Source: CAD feature listing. Evaluate the final solid. Frame: model axes, mm. Round coordinates to 2 decimals unless told otherwise and drop trailing zeros. Order: outer loops, then holes, each group sorted by start corner. A loop starts at its lowest first (then second) coordinate and runs counter-clockwise, first axis right, second up. Notation, with made-up numbers: (73, 17.25) -> (114, 17.25) arc R21 ccw to (114, 27.25) -> close; hole circle Ø10 at (61, 25). An arc over 180 degrees is marked (long way). Use a Markdown table: item, result. Add a question column.
```python
from build123d import *

# Parameters (mm, degrees)
F0_W     = 300
F0_H     = 10
F1_DEPTH = 100
F2_R     = 2.75
F2_R_2   = 4.25
F3_DEPTH = 10.001
F4_R     = 2.75
F5_DEPTH = 10.001
F6_SIZE  = 0.5


with BuildPart() as f1:
    # F0 (on Right) → F1 (new body)
    with BuildSketch(Plane.YZ):
        with Locations((-150, 5)):
            Rectangle(F0_W, F0_H)
    extrude(amount=F1_DEPTH)

    # F2 (on face) → F3 (cut, through all)
    with BuildSketch(Plane.XY.offset(10)):
        with Locations((60.5, -83)):
            Circle(F2_R)
        with Locations((39.5, -83)):
            Circle(F2_R)
        with Locations((39.5, -217)):
            Circle(F2_R)
        with Locations((60.5, -217)):
            Circle(F2_R)
        with Locations((15, -215)):
            Circle(F2_R_2)
        with Locations((15, -195)):
            Circle(F2_R_2)
        with Locations((15, -83)):
            Circle(F2_R_2)
        with Locations((15, -63)):
            Circle(F2_R_2)
        with Locations((15, -23)):
            Circle(F2_R_2)
    extrude(amount=-F3_DEPTH, mode=Mode.SUBTRACT)

    # F4 (on face) → F5 (cut, through all)
    with BuildSketch(Plane.XY.offset(10)):
        with Locations((80, -193)):
            Circle(F4_R)
        with Locations((80, -173)):
            Circle(F4_R)
        with Locations((80, -133)):
            Circle(F4_R)
        with Locations((80, -113)):
            Circle(F4_R)
        with Locations((80, -73)):
            Circle(F4_R)
        with Locations((80, -53)):
            Circle(F4_R)
        with Locations((80, -33)):
            Circle(F4_R)
    extrude(amount=-F5_DEPTH, mode=Mode.SUBTRACT)

    # F6
    f6_edges = [f1.edges().sort_by_distance(p)[0] for p in [
        (77.25, -53, 10),
        (82.75, -53, 5),
        (77.25, -53, 0),
        (77.25, -73, 10),
        (82.75, -73, 5),
        (77.25, -73, 0),
        (77.25, -113, 10),
        (82.75, -113, 5),
        (77.25, -113, 0),
        (77.25, -133, 10),
        (82.75, -133, 5),
        (77.25, -133, 0),
        (77.25, -173, 10),
        (82.75, -173, 5),
        (77.25, -173, 0),
        (77.25, -193, 10),
        (82.75, -193, 5),
        (77.25, -193, 0),
        (77.25, -33, 10),
        (82.75, -33, 5),
        (77.25, -33, 0),
    ]]
    chamfer(f6_edges, length=F6_SIZE)


solid = f1.part
```
1) Section B-B on z = 4.5. Count the separate pieces of the cut face and the enclosed holes in it, then the cut area to 3 significant figures.
2) Line query: probe 1 along Y at (x, z) = (15, 5); probe 2 along Y at (x, z) = (40, 0.5); probe 3 along Y at (x, z) = (59, 1.25). Output: solid intervals per line, ascending. Write a range as from..to.
3) Draft query along Y for faces 1 (the flat face through (49, 0, 5)), 2 (the flat face through (49, -152, 10)), 3 (the cylindrical face through (77.818, -174.673, 5.063)), 4 (the flat face through (49, -300, 5)). Return one class per face: pulls with the +Y half, pulls with the -Y half, needs draft (parallel to the pull), parting line crosses it, or undercut.
4) Section C-C on y = -113. Output: boundary loops of the cut face in (x, z).
5) Section A-A on y = -23. Output: boundary loops of the cut face in (x, z), then the cut area to 3 significant figures.
Conclusion:
| question | item | result |
|---|---|---|
| 1 | separate pieces | 1 |
| 1 | enclosed holes | 16 |
| 1 | area | 29,500 mm^2 |
| 2 | probe 1 | y = -300..-219.25, -210.75..-199.25, -190.75..-87.25, -78.75..-67.25, -58.75..-27.25, -18.75..0 |
| 2 | probe 2 | y = -300..-219.7, -214.3..-85.7, -80.3..0 |
| 2 | probe 3 | y = -300..-219.3, -214.7..-85.3, -80.7..0 |
| 3 | face 1 | pulls with the +Y half |
| 3 | face 2 | needs draft |
| 3 | face 3 | undercut |
| 3 | face 4 | pulls with the -Y half |
| 4 | outline | (0, 0) -> (76.75, 0) -> (77.25, 0.5) -> (77.25, 9.5) -> (76.75, 10) -> (0, 10) -> close; (82.75, 0.5) -> (83.25, 0) -> (100, 0) -> (100, 10) -> (83.25, 10) -> (82.75, 9.5) -> close |
| 5 | outline | (0, 0) -> (10.75, 0) -> (10.75, 10) -> (0, 10) -> close; (19.25, 0) -> (100, 0) -> (100, 10) -> (19.25, 10) -> close |
| 5 | area | 915 mm^2 |
